Geometry check sheet. Reference: the model listing, model coordinates, mm. Face numbers are marked on the shaded views. Round coordinates to 2 decimals unless told otherwise and drop trailing zeros. Order: outer loops, then holes, each group sorted by start corner. A loop starts at its lowest first (then second) coordinate and runs counter-clockwise, first axis right, second up.
(1) Thickness scan on L1, parallel to Y at x = 0, z = -3.55; L2, parallel to Y at x = 3, z = -2. Record the ranges inside material, lowest first.
(2) Cross-section at D-D on z = -3. Enter the section's corners in (x, y), and give its area (3 significant figures).
(3) Gauge pin test, flat ends, axial feed: P1, Ø5, axis at x = 2, y = 0.5, coming from the -Z side; P2, Ø1.5, axis at y = -4.5, z = -1, coming from the +X side; P3, Ø0.6, axis at x = 0.5, y = -5.5, coming from the +Z side. Record the tip position at first contact, or that the pin passes through.
(4) Draft check along Y on the marked faces 1, 2, 3 and 4. Enter one of: pulls with the +Y half, pulls with the -Y half, needs draft (parallel to the pull), parting line crosses it, or undercut.
(5) Cross-section at A-A on x = 0. Enter the section's corners in (y, z), and give its area (3 significant figures).
(6) Cross-section at C-C on z = -0.5. Enter the section's corners in (x, y), and give its area (3 significant figures).
(7) Cross-section at B-B on y = 0. Enter the section's corners in (x, z), and give its area (3 significant figures).
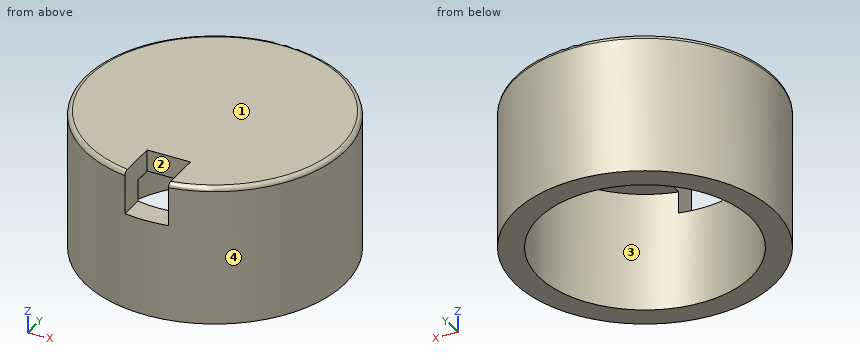
from build123d import *

# Parameters (mm, degrees)
SKETCH_1_R          = 6
SKETCH_1_R_2        = 4.9
EXTRUDE_1_DEPTH     = 6.5
SKETCH_1_2_R        = 4.9
EXTRUDE_2_DEPTH     = 1
FILLET_2_R          = 0.2
SKETCH_8_W          = 2
SKETCH_8_H          = 2
CUT_EXTRUDE_2_DEPTH = 2


with BuildPart() as part:
    # Sketch 1 → Extrude 1 (new body)
    with BuildSketch(Plane.XY):
        Circle(SKETCH_1_R)
        Circle(SKETCH_1_R_2, mode=Mode.SUBTRACT)
    extrude(amount=-EXTRUDE_1_DEPTH)

    # Sketch 1_2 → Extrude 2 (add)
    with BuildSketch(Plane.XY):
        Circle(SKETCH_1_2_R)
    extrude(amount=-EXTRUDE_2_DEPTH)

    # Fillet 2
    fillet_2_edges = [part.edges().sort_by_distance(p)[0] for p in [
        (-6, 0, 0),
    ]]
    fillet(fillet_2_edges, radius=FILLET_2_R)

    # Sketch 8 → Cut-Extrude 2 (cut)
    with BuildSketch(Plane(origin=(0, -6, 0), x_dir=(1, 0, 0), z_dir=(0, 1, 0))):
        with Locations((0, 1)):
            Rectangle(SKETCH_8_W, SKETCH_8_H)
    extrude(amount=CUT_EXTRUDE_2_DEPTH, mode=Mode.SUBTRACT)


solid = part.part
Found:
1. L1: y = -6 to -4.9, 4.9 to 6
1. L2: y = -5.2 to -3.87, 3.87 to 5.2
2. outline: circle Ø12 at (0, 0); hole circle Ø9.8 at (0, 0)
2. area: 37.7 mm2
3. P1: stops at z = -1
3. P2: stops at x = 4.68
3. P3: stops at z = -2
4. face 1: needs draft
4. face 2: pulls with the -Y half
4. face 3: undercut
4. face 4: parting line crosses it
5. outline: (-6, -6.5) - (-4.9, -6.5) - (-4.9, -2) - (-6, -2) - close; (-4, -1) - (4.9, -1) - (4.9, -6.5) - (6, -6.5) - (6, -0.2) arc R0.2 ccw to (5.8, 0) - (-4, 0) - close
5. area: 21.0 mm2
6. outline: (-1, -5.92) - (-1, -4) - (1, -4) - (1, -5.92) arc R6 ccw (long way) to start
6. area: 109 mm2
7. outline: (-6, -6.5) - (-4.9, -6.5) - (-4.9, -1) - (4.9, -1) - (4.9, -6.5) - (6, -6.5) - (6, -0.2) arc R0.2 ccw to (5.8, 0) - (-5.8, 0) arc R0.2 ccw to (-6, -0.2) - close
7. area: 24.1 mm2
